```python
from build123d import *

# Parameters (mm, degrees)
F0_R      = 12.7368274584
F1_DEPTH  = 5.08
F2_R      = 5.07999
F3_R      = 11.9321398377
F4_DEPTH  = 13.97
F5_R      = 5.08
F6_R      = 6.5535099449
F7_DEPTH  = 24.13
F8_DEPTH  = 27.94
F8_FACE_R = 6.5535099449
F9_DEPTH  = 12.7
F9_TAPER  = -15
F11_DEPTH = 25.4


# Not quite as in the source:
# - a fillet or chamfer is up to 0.001 mm smaller than in the source, because OpenCascade refuses the exact size


with BuildPart() as f1:
    # F0 (on Top) → F1 (new body)
    with BuildSketch(Plane.XY):
        Circle(F0_R)
    extrude(amount=F1_DEPTH)

    # F2 (radius 5.08 in the source; OpenCascade refuses exactly that, so slightly less here)
    f2_edges = [f1.edges().sort_by_distance(p)[0] for p in [
        (-12.736827, 0, 5.08),
    ]]
    fillet(f2_edges, radius=F2_R)

    # F3 (on Top) → F4 (join)
    with BuildSketch(Plane.XY):
        Circle(F3_R)
    extrude(amount=F4_DEPTH)

    # F5
    f5_edges = [f1.edges().sort_by_distance(p)[0] for p in [
        (-11.93214, 0, 2.743746),
        (11.93214, 0, 8.356873),
        (-11.93214, 0, 13.97),
    ]]
    fillet(f5_edges, radius=F5_R)

    # F6 (on Top) → F7 (join)
    with BuildSketch(Plane.XY):
        Circle(F6_R)
    extrude(amount=F7_DEPTH)

    # F8 (add): a face of the model
    f8_faces = [f1.faces().sort_by_distance(p)[0] for p in [
        (0, 0, 24.13),
    ]]
    extrude(f8_faces, amount=F8_DEPTH)

    # F8_face (on face) → F9 (join)
    with BuildSketch(Plane.XY.offset(52.07)):
        Circle(F8_FACE_R)
    extrude(amount=F9_DEPTH, taper=F9_TAPER)

    # F10 (on face) → F11 (cut)
    with BuildSketch(Plane.XY.offset(64.77)):
        with BuildLine():
            Line((3.9382930845, -5.420595399), (3.9382930845, -9.1444538754))
            ThreePointArc((3.9382930845, -9.1444538754), (5.852263109, -8.0549491371), (7.4798929542, -6.5713309529))
            Line((7.4798929542, -6.5713309529), (3.9382930845, -5.420595399))
        make_face()
        with BuildLine():
            Line((8.5611211624, 5.0831479952), (6.3722920684, 2.0704832032))
            Line((6.3722920684, 2.0704832032), (9.9138919381, 0.9197476493))
            ThreePointArc((9.9138919381, 0.9197476493), (9.4691606215, 3.0767167927), (8.5611211624, 5.0831479952))
        make_face()
        with BuildLine():
            Line((-2.188829094, 9.7128891837), (0, 6.7002243917))
            Line((0, 6.7002243917), (2.188829094, 9.7128891837))
            ThreePointArc((2.188829094, 9.7128891837), (0, 9.9564646887), (-2.188829094, 9.7128891837))
        make_face()
        with BuildLine():
            ThreePointArc((-8.5611211624, 5.0831479952), (-9.4691606215, 3.0767167927), (-9.9138919381, 0.9197476493))
            Line((-9.9138919381, 0.9197476493), (-6.3722920684, 2.0704832032))
            Line((-6.3722920684, 2.0704832032), (-8.5611211624, 5.0831479952))
        make_face()
        with BuildLine():
            ThreePointArc((-7.4798929542, -6.5713309529), (-5.852263109, -8.0549491371), (-3.9382930845, -9.1444538754))
            Line((-3.9382930845, -9.1444538754), (-3.9382930845, -5.420595399))
            Line((-3.9382930845, -5.420595399), (-7.4798929542, -6.5713309529))
        make_face()
    extrude(amount=-F11_DEPTH, mode=Mode.SUBTRACT)


solid = f1.part
```
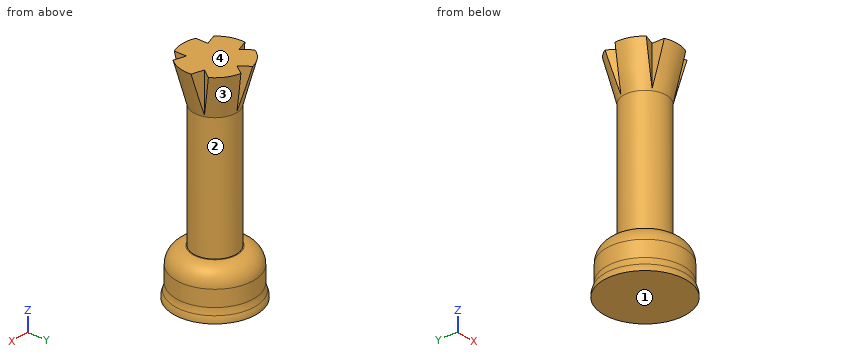
Verification items for the finished model (mm, model axes). Face numbers are marked on the shaded views. Coordinates: 2 decimals unless noted, no trailing zeros. Loops run counter-clockwise (first coordinate to the right, second up) from the corner with the lowest first, then second, coordinate; pieces in that order, holes last. Notation, with made-up numbers: (19, 21.25) -> (31, 21.25) arc R19 ccw to (31, 48.25) -> close; hole circle Ø8 at (-3.5, 64.25). An arc over 180 degrees is marked (long way). Answer in a Markdown table with one row per item. Add a question column.
1. Section check A-A, the plane z = 32.5. Enter the section's corners in (x, y).
2. Section check B-B, the plane y = 8.75. Give the number of separate pieces and of enclosed holes in the cut face, then the cut area to 3 significant figures.
3. Material ranges on probe 1 along X at (y, z) = (1.5, 43.5); probe 2 along X at (y, z) = (2.5, 55.5), recorded low to high. Write a range as [from, to].
4. Section check C-C, the plane z = 5.5. Enter the section's corners in (x, y), then the cut area to 3 significant figures.
5. Depth check by flat-ended pin: P1, Ø5, axis at x = -0.5, z = 25.5, coming from the +Y side; P2, Ø4, axis at x = -6.5, z = 16, coming from the +Y side; P3, Ø2, axis at x = -1, z = 9.5, coming from the +Y side; P4, Ø3, axis at x = -9, z = 37, coming from the +Y side. Enter the tip coordinate at first touch or a pass-through.
6. Draft check along Z on the marked faces 1, 2, 3 and 4. Enter one of: +Z half, -Z half, draft (parallel to the pull), parting line (faces both ways), or undercut.
Derived:
| question | item | result |
|---|---|---|
| 1 | outline | circle Ø13.11 at (0, 0) |
| 2 | separate pieces | 3 |
| 2 | enclosed holes | 0 |
| 2 | area | 226 mm² |
| 3 | probe 1 | x = [-6.38, 6.38] |
| 3 | probe 2 | x = [-6.68, 6.68] |
| 4 | outline | circle Ø23.86 at (0, 0) |
| 4 | area | 447 mm² |
| 5 | P1 | stops at y = 6.55 |
| 5 | P2 | stops at y = 4.76 |
| 5 | P3 | stops at y = 11.93 |
| 5 | P4 | passes through |
| 6 | face 1 | -Z half |
| 6 | face 2 | undercut |
| 6 | face 3 | undercut |
| 6 | face 4 | +Z half |
